Geometry check sheet. Reference: the model listing, model coordinates, mm. A direction names the side the tool comes from. Round coordinates to 2 decimals unless told otherwise and drop trailing zeros. Order: outer loops, then holes, each group sorted by start corner. A loop starts at its lowest first (then second) coordinate and runs counter-clockwise, first axis right, second up.
Autodesk Inventor part; units mm, degrees
ref_plane "YZ Plane" through (0, 0, 0) normal (1, 0, 0) x (0, 1, 0)
ref_plane "XZ Plane" through (0, 0, 0) normal (0, 1, 0) x (-1, 0, 0)
ref_plane "XY Plane" through (0, 0, 0) normal (0, 0, 1) x (1, 0, 0)
sketch "Sketch1" plane through (0, 0, 0) normal (0, 0, 1) x (1, 0, 0)
  line L0 (12.7, -25.4) -> (-12.7, -25.4)
  line L1 (-12.7, -25.4) -> (-12.7, 25.4)
  line L2 (-12.7, 25.4) -> (12.7, 25.4)
  line L3 (12.7, 25.4) -> (12.7, -25.4)
  line L4 (12.7, -25.4) -> (-12.7, 25.4) construction
  line L5 (-12.7, -25.4) -> (12.7, 25.4) construction
  line L6 (10.16, 22.86) -> (-10.16, 22.86)
  line L7 (-10.16, 22.86) -> (-10.16, -22.86)
  line L8 (-10.16, -22.86) -> (10.16, -22.86)
  line L9 (10.16, -22.86) -> (10.16, 22.86)
  point P0 (0, 0)
  dimension "d0" = 25.4
  dimension "d1" = 50.8
  dimension "d2" = 2.54
extrude "Extrusion1" add sketch "Sketch1" along normal mid plane 406.4
sketch "Sketch2" plane through (-12.7, 25.4, 203.2) normal (0, 1, 0) x (1, 0, 0)
  point P0 (12.7, 203.2)
  point P1 (12.7, 215.9)
  point P2 (12.7, 190.5)
  dimension "HoleOffset" = 12.7
  dimension "d6" = 12.7
hole "Hole1" at (0, 25.4, -12.7) at (0, 25.4, 12.7) direction (0, -1, 0) diameter 4.1656 end through all
pattern_linear "Rectangular Pattern1" count 31 spacing 50.8 along (0, 0, 1) of "Hole1" first direction both ways yes
properties part number "Base Frame Side Rail" material "Aluminum 6061"
(1) Set-up check for faces 1 (the flat face through (10.16, 0, -3)), 2 (the flat face through (12.7, 0, -3)): record each of +Z, -Z, +X, -X, +Y, -Y from which the full face is reachable in a straight line by a thin tool's end or side.
Returned:
face 1: +Z, -Z
face 2: +Z, -Z, +X, +Y, -Y
(2) Sectioned sample at B-B, the plane x = 6.25. Record the cut outline in (y, z).
Returned:
outline: (-25.4, -203.2) - (-22.86, -203.2) - (-22.86, 203.2) - (-25.4, 203.2) - close; (22.86, -203.2) - (25.4, -203.2) - (25.4, 203.2) - (22.86, 203.2) - close
(3) Sectioned sample at A-A, the plane y = -16.5. Record the cut outline in (x, z), and give its area (3 significant figures).
Returned:
outline: (-12.7, -203.2) - (-10.16, -203.2) - (-10.16, 203.2) - (-12.7, 203.2) - close; (10.16, -203.2) - (12.7, -203.2) - (12.7, 203.2) - (10.16, 203.2) - close
area: 2,060 mm2
(4) Draft check along Y on faces 3 (the flat face through (0, -25.4, -3)), 4 (the flat face through (0, -22.86, -3)), 5 (the flat face through (0, 22.86, -3)), 6 (the flat face through (-10.4, 2, -203.2)). Enter one of: released by +Y, released by -Y, zero draft, split by the parting line, or undercut.
Returned:
face 3: released by -Y
face 4: undercut
face 5: undercut
face 6: zero draft
(5) Sectioned sample at C-C, the plane z = 78.5. Record the cut outline in (x, y), and give its area (3 significant figures).
Returned:
outline: (-12.7, -25.4) - (12.7, -25.4) - (12.7, 25.4) - (-12.7, 25.4) - close; hole (-10.16, -22.86) - (10.16, -22.86) - (10.16, 22.86) - (-10.16, 22.86) - close
area: 361 mm2
(6) Material ranges on line 1 (X direction, y = 1, z = 112); line 2 (X direction, y = -24.8, z = -12.7); line 3 (Y direction, x = -7, z = -73), recorded low to high.
Returned:
line 1: x = -12.7 to -10.16, 10.16 to 12.7
line 2: x = -12.7 to -2.08, 2.08 to 12.7
line 3: y = -25.4 to -22.86, 22.86 to 25.4
